CAD build for the part. Positions are in the model's coordinates, mm. Face numbers are marked on the shaded views. A direction names the side the tool comes from. Coordinates: 2 decimals unless noted, no trailing zeros. Write each loop counter-clockwise with the first axis right and the second up, starting at its lowest first coordinate (ties: lowest second). Pieces come first, ordered by that corner, then holes. Notation, with made-up numbers: M -31.75,64.5 L -26.75,64.5 A28 ccw -26.75,98.5 Z; hole C 71,-6 d2. An arc over 180 degrees is marked long. Answer as CSV lines item,"result". Start each with the question number.
```python
from build123d import *

# Parameters (mm, degrees)
BOSS_EXTRUDE1_DEPTH            = 60
HOLE_FOR_M5_300_SC_NUTS_SP_1_D = 10
HOLE_FOR_M5_300_SC_NUTS_SP_2_D = 3.5


with BuildPart() as part:
    # Sketch1 → Boss-Extrude1 (new body)
    with BuildSketch(Plane.XY):
        Polygon((-7.897485035, 31.347562808), (-7.897485035, 2.347562808), (14.102514965, 2.347562808), (14.102514965, -0.652437192), (-10.897485035, -0.652437192), (-10.897485035, 31.347562808), align=None)
    extrude(amount=BOSS_EXTRUDE1_DEPTH)

    # Hole for M5 300® SC Nuts (SP)1 (through all)
    with Locations(Plane(origin=(-7.897485035, 0, 0), x_dir=(0, 0, -1), z_dir=(1, 0, 0))):
        with Locations((-30, 22.347562808)):
            Hole(HOLE_FOR_M5_300_SC_NUTS_SP_1_D / 2)

    # Hole for M5 300® SC Nuts (SP)2 (through all)
    with Locations(Plane(origin=(-7.897485035, 0, 0), x_dir=(0, 0, -1), z_dir=(1, 0, 0))):
        with Locations((-22, 22.347562808), (-38, 22.347562808), (-30, 14.347562808)):
            Hole(HOLE_FOR_M5_300_SC_NUTS_SP_2_D / 2)


solid = part.part
```
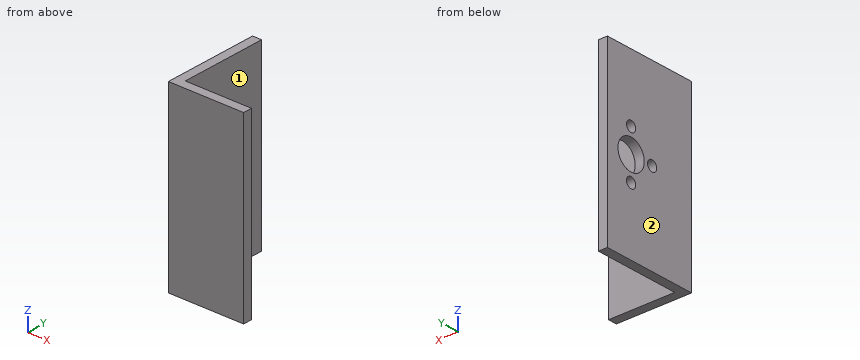
1) Band-saw the part on C-C, the plane z = 30. List the corners of the cut face in (x, y), plus the area to 4 significant figures.
2) Band-saw the part on B-B, the plane y = 23.5. List the corners of the cut face in (x, z), plus the area to 3 significant figures.
3) Band-saw the part on D-D, the plane y = 19. List the corners of the cut face in (x, z).
4) Band-saw the part on A-A, the plane z = 22. List the corners of the cut face in (x, y).
5) Tool access for the marked faces 1 and 2: list every direction of +Z, -Z, +X, -X, +Y, -Y with a clear straight run to the whole face (end or side of a thin tool).
6) Probe L1, parallel to Y at x = -9.55, z = 30; L2, parallel to Z at x = -9.25, y = 22.5; L3, parallel to Y at x = -8.9, z = 38. List the from-to ranges inside material, lowest first. Write a range as [from, to].
7) Pin check, flat tips, straight feed: P1, Ø3, axis at y = 22.35, z = 38, coming from the -X side; P2, Ø16, axis at y = 22.35, z = 30, coming from the +X side; P3, Ø1, axis at x = 5, z = 27, coming from the +Y side. Stop position of each tip, or through.
Result sheet:
1,outline,"M -10.9,-0.65 L 14.1,-0.65 L 14.1,2.35 L -7.9,2.35 L -7.9,12.6 L -10.9,12.6 Z; M -10.9,16.1 L -7.9,16.1 L -7.9,17.35 L -10.9,17.35 Z; M -10.9,27.35 L -7.9,27.35 L -7.9,31.35 L -10.9,31.35 Z"
1,area,"121.5 mm²"
2,outline,"M -10.9,0 L -7.9,0 L -7.9,20.68 L -10.9,20.68 Z; M -10.9,23.32 L -7.9,23.32 L -7.9,25.13 L -10.9,25.13 Z; M -10.9,34.87 L -7.9,34.87 L -7.9,36.68 L -10.9,36.68 Z; M -10.9,39.32 L -7.9,39.32 L -7.9,60 L -10.9,60 Z"
2,area,"135 mm²"
3,outline,"M -10.9,0 L -7.9,0 L -7.9,26.29 L -10.9,26.29 Z; M -10.9,33.71 L -7.9,33.71 L -7.9,60 L -10.9,60 Z"
4,outline,"M -10.9,-0.65 L 14.1,-0.65 L 14.1,2.35 L -7.9,2.35 L -7.9,20.6 L -10.9,20.6 Z; M -10.9,24.1 L -7.9,24.1 L -7.9,31.35 L -10.9,31.35 Z"
5,face 1,"+Z, -Z, +X, +Y"
5,face 2,"+Z, -Z, -X, +Y, -Y"
6,L1,"y = [-0.65, 12.6], [16.1, 17.35], [27.35, 31.35]"
6,L2,"z = [0, 20.26], [23.74, 25], [35, 36.26], [39.74, 60]"
6,L3,"y = [-0.65, 20.6], [24.1, 31.35]"
7,P1,"passes through"
7,P2,"stops at x = -7.9"
7,P3,"stops at y = 2.35"
